from build123d import *

# Parameters (mm, degrees)
F1_DEPTH = 25.4
F2_R     = 5.08
F3_R     = 5.08


with BuildPart() as f1:
    # F0 (on Top) → F1 (new body)
    with BuildSketch(Plane.XY):
        Polygon((52.649982, 33.518303), (-43.856528, -18.63311), (33.346899, -18.63311), align=None)
    extrude(amount=F1_DEPTH)

    # F2
    f2_edges = [f1.edges().sort_by_distance(p)[0] for p in [
        (33.346899, -18.63311, 12.7),
    ]]
    fillet(f2_edges, radius=F2_R)

    # F3
    f3_edges = [f1.edges().sort_by_distance(p)[0] for p in [
        (-7.023078, -18.63311, 25.4),
        (32.712825, -17.722303, 25.4),
        (4.396727, 7.442596, 25.4),
        (43.612241, 9.10091, 25.4),
    ]]
    fillet(f3_edges, radius=F3_R)


solid = f1.part
Could you check a few things on this model? Use its own coordinates, in mm. Coordinates: 2 decimals unless noted, no trailing zeros. Order: outer loops, then holes, each group sorted by start corner. A loop starts at its lowest first (then second) coordinate and runs counter-clockwise, first axis right, second up. Notation, with made-up numbers: (83.5, 16.25) -> (108.5, 16.25) arc R10 ccw to (108.5, 22.25) -> close; hole circle Ø2 at (31, -8). An arc over 180 degrees is marked (long way). One line per question, with ' | ' between items.
Q1. If I drill on L1, parallel to X at y = 17, z = 8.5; L2, parallel to X at y = -1.5, z = 9.75; L3, parallel to Z at x = -22, y = -10, over which ranges is the centre line in solid material (lowest first)?
Return value:
L1: 22.08 to 46.54 | L2: -12.15 to 39.69 | L3: 0 to 24.86
Q2. Imagine slicing it at B-B on z = 21.75. Please give me the cut outline in (x, y).
Return value:
outline: (-43.04, -18.43) -> (29.81, -18.43) arc R4.87 ccw to (34.38, -15.25) -> (52.27, 33.08) -> close
Q3. Imagine slicing it at A-A on z = 12. Please give me the cut outline in (x, y), and give its area (3 significant figures).
Return value:
outline: (-43.86, -18.63) -> (29.81, -18.63) arc R5.08 ccw to (34.57, -15.32) -> (52.65, 33.52) -> close | area: 2,010 mm²
Q4. I'm going to push flat-ended pins straight in: P1, Ø1.5, axis at y = -9.5, z = 11, coming from the +X side (3 decimals); P2, Ø2, axis at x = -9, z = 21, coming from the -Y side; P3, Ø3, axis at y = -11, z = 19, coming from the +X side; P4, Ø10, axis at x = 30.5, z = 18.5, coming from the +Y side. Where does each tip first touch, or does it pass through?
Return value:
P1: x = 37.005 | P2: y = -18.63 | P3: x = 36.73 | P4: y = 24.25
